Geometry check sheet. Reference: the model listing, model coordinates, mm. Coordinates: 2 decimals unless noted, no trailing zeros. Write each loop counter-clockwise with the first axis right and the second up, starting at its lowest first coordinate (ties: lowest second). Pieces come first, ordered by that corner, then holes. Notation, with made-up numbers: M 84,17 L 131,17 A7 ccw 131,29 Z; hole C 34,86.5 d2. An arc over 180 degrees is marked long. Write item = value, one per line. Start each with the question number.
```python
from build123d import *

# Parameters (mm, degrees)
SKETCH1_W           = 76.2
SKETCH1_H           = 101.6
BOSS_EXTRUDE1_DEPTH = 25.4
FILLET1_R           = 6.35
CUT_EXTRUDE1_DEPTH  = 6.35
SKETCH4_W           = 6.834349176
SKETCH4_H           = 11.846205237
BOSS_EXTRUDE2_DEPTH = 2.54
FILLET2_R           = 0.762


with BuildPart() as part:
    # Sketch1 → Boss-Extrude1 (new body)
    with BuildSketch(Plane(origin=(0, 0, 0), x_dir=(1, 0, 0), z_dir=(0, 1, 0))):
        Rectangle(SKETCH1_W, SKETCH1_H)
    extrude(amount=BOSS_EXTRUDE1_DEPTH)

    # Fillet1
    fillet1_edges = [part.edges().sort_by_distance(p)[0] for p in [
        (38.1, 25.4, 0),
        (0, 25.4, -50.8),
        (-38.1, 25.4, 0),
        (0, 0, -50.8),
        (38.1, 0, 0),
        (0, 0, 50.8),
        (-38.1, 0, 0),
        (0, 25.4, 50.8),
        (-38.1, 12.7, -50.8),
        (38.1, 12.7, -50.8),
        (38.1, 12.7, 50.8),
        (-38.1, 12.7, 50.8),
    ]]
    fillet(fillet1_edges, radius=FILLET1_R)

    # Sketch3 → Cut-Extrude1 (cut)
    with BuildSketch(Plane(origin=(0, 25.4, 0), x_dir=(1, 0, 0), z_dir=(0, 1, 0))):
        with BuildLine():
            Line((15.491191464, -37.475014645), (-15.491191464, -37.475014645))
            ThreePointArc((-15.491191464, -37.475014645), (-17.883213675, -35.082992433), (-15.491191464, -32.690970222))
            Line((-15.491191464, -32.690970222), (15.491191464, -32.690970222))
            ThreePointArc((15.491191464, -32.690970222), (17.883213675, -35.082992433), (15.491191464, -37.475014645))
        make_face()
        with BuildLine():
            Line((15.491191464, -27.315014645), (-15.491191464, -27.315014645))
            ThreePointArc((-15.491191464, -27.315014645), (-17.883213675, -24.922992433), (-15.491191464, -22.530970222))
            Line((-15.491191464, -22.530970222), (15.491191464, -22.530970222))
            ThreePointArc((15.491191464, -22.530970222), (17.883213675, -24.922992433), (15.491191464, -27.315014645))
        make_face()
        with BuildLine():
            Line((15.491191464, -17.155014645), (-15.491191464, -17.155014645))
            ThreePointArc((-15.491191464, -17.155014645), (-17.883213675, -14.762992433), (-15.491191464, -12.370970222))
            Line((-15.491191464, -12.370970222), (15.491191464, -12.370970222))
            ThreePointArc((15.491191464, -12.370970222), (17.883213675, -14.762992433), (15.491191464, -17.155014645))
        make_face()
    extrude(amount=-CUT_EXTRUDE1_DEPTH, mode=Mode.SUBTRACT)

    # Sketch4 → Boss-Extrude2 (add)
    with BuildSketch(Plane(origin=(0, 25.4, 0), x_dir=(1, 0, 0), z_dir=(0, 1, 0))):
        with Locations((0, 29.615513094)):
            Rectangle(SKETCH4_W, SKETCH4_H)
    extrude(amount=BOSS_EXTRUDE2_DEPTH)

    # Fillet2
    fillet2_edges = [part.edges().sort_by_distance(p)[0] for p in [
        (-3.417174588, 26.67, -35.538615712),
        (-3.417174588, 26.67, -23.692410475),
        (3.417174588, 26.67, -23.692410475),
        (3.417174588, 26.67, -35.538615712),
    ]]
    fillet(fillet2_edges, radius=FILLET2_R)


solid = part.part
```
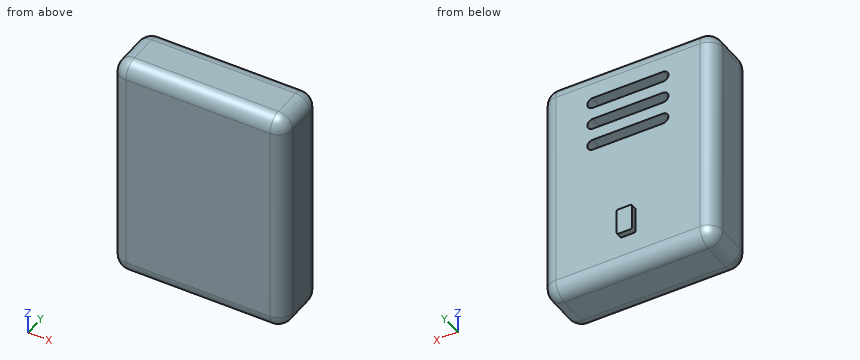
Q1. Cross-section at C-C on x = -10. Enter the section's corners in (y, z), and give its area (3 significant figures).
Q2. Cross-section at A-A on z = -18. Enter the section's corners in (x, y), and give its area (3 significant figures).
Q3. Cross-section at B-B on y = 24.25. Enter the section's corners in (x, z), and give its area (3 significant figures).
Q4. Gauge pin test, flat ends, axial feed: pin 1 (1.9 mm diameter, centred on x = 1, y = 23, fed in from -Z); pin 2 (1.9 mm diameter, centred on x = 3.5, y = 23, fed in from +Z); pin 3 (4 mm diameter, centred on x = -3.5, z = 25.5, fed in from +Y). Record the tip position at first contact, or that the pin passes through.
Q5. Cross-section at D-D on x = 27.5. Enter the section's corners in (y, z), and give its area (3 significant figures).
Q6. Scan lines: L1, parallel to Y at x = 8.5, z = -16.5; L2, parallel to Y at x = 12, z = 37; L3, parallel to Z at x = 0.5, y = 22. Record each from-to range of solid material in increasing order.
Values found:
q1.outline = M 0,-44.45 A6.35 ccw 6.35,-50.8 L 19.05,-50.8 A6.35 ccw 25.4,-44.45 L 25.4,12.37 L 19.05,12.37 L 19.05,17.16 L 25.4,17.16 L 25.4,22.53 L 19.05,22.53 L 19.05,27.32 L 25.4,27.32 L 25.4,32.69 L 19.05,32.69 L 19.05,37.48 L 25.4,37.48 L 25.4,44.45 A6.35 ccw 19.05,50.8 L 6.35,50.8 A6.35 ccw 0,44.45 Z
q1.area = 2,450 mm²
q2.outline = M -38.1,6.35 A6.35 ccw -31.75,0 L 31.75,0 A6.35 ccw 38.1,6.35 L 38.1,19.05 A6.35 ccw 31.75,25.4 L -31.75,25.4 A6.35 ccw -38.1,19.05 Z
q2.area = 1,900 mm²
q3.outline = M -35.39,-44.45 A3.64 ccw -31.75,-48.09 L 31.75,-48.09 A3.64 ccw 35.39,-44.45 L 35.39,44.45 A3.64 ccw 31.75,48.09 L -31.75,48.09 A3.64 ccw -35.39,44.45 Z; hole M -15.49,12.37 L 15.49,12.37 A2.39 ccw 15.49,17.16 L -15.49,17.16 A2.39 ccw Z; hole M -15.49,22.53 L 15.49,22.53 A2.39 ccw 15.49,27.32 L -15.49,27.32 A2.39 ccw Z; hole M -15.49,32.69 L 15.49,32.69 A2.39 ccw 15.49,37.48 L -15.49,37.48 A2.39 ccw Z
q3.area = 6,300 mm²
q4.pin_1 = -50.05
q4.pin_2 = 50.05
q4.pin_3 = 25.4
q5.outline = M 0,-44.45 A6.35 ccw 6.35,-50.8 L 19.05,-50.8 A6.35 ccw 25.4,-44.45 L 25.4,44.45 A6.35 ccw 19.05,50.8 L 6.35,50.8 A6.35 ccw 0,44.45 Z
q5.area = 2,550 mm²
q6.L1 = 0 to 25.4
q6.L2 = 0 to 19.05
q6.L3 = -50.07 to 12.37, 17.16 to 22.53, 27.32 to 32.69, 37.48 to 50.07
